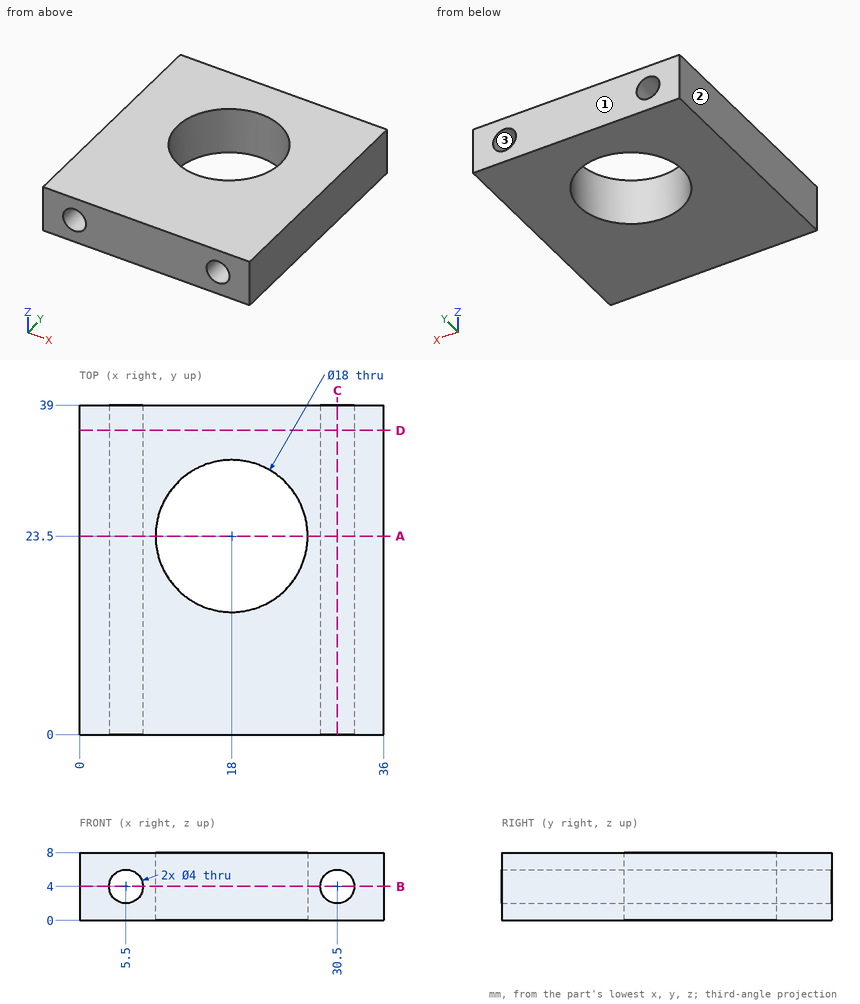
Answer from the drawing. Dimensions are ordinates in mm from the lowest x, y and z of the part. Coordinates: 2 decimals unless noted, no trailing zeros. Order: outer loops, then holes, each group sorted by start corner. A loop starts at its lowest first (then second) coordinate and runs counter-clockwise, first axis right, second up. Notation, with made-up numbers: (19.5, 31.25) - (27.5, 31.25) arc R22 cw to (27.5, 67.25) - close; hole circle Ø4 at (-10, 64.5). An arc over 180 degrees is marked (long way). Answer as a JSON object with one key per item and string values. Group by question number.
Item 1: Section D-D (y = 36) is taken. Give the vertices of the cut face in (x, z).
Item 2: Flat-ended cylindrical pins translate along their axes: P1, Ø1.5, axis at y = 31, z = 5, coming from the -X side; P2, Ø14.5, axis at x = 18, y = 23.5, coming from the +Z side. Find the tip coordinate at first contact, or state that the pin passes through.
Item 3: The mould has two halves that part along X. Classify the marked faces 1, 2 and 3: +X half, -X half, draft (parallel to the pull), parting line (faces both ways), or undercut.
Item 4: Section C-C (x = 30.5) is taken. Give the vertices of the cut face in (y, z).
Item 5: Consider probe 1 along X at (y, z) = (35.5, 4); probe 2 along X at (y, z) = (31.5, 4); probe 3 along X at (y, z) = (30.5, 4). Determine where each line is inside the solid, lowest interval first. Write a range as from..to.
Item 6: Section B-B (z = 4) is taken. Give the vertices of the cut face in (x, y), plus the area to 3 significant figures.
Item 7: Section A-A (y = 23.5) is taken. Give the vertices of the cut face in (x, z), plus the area to 3 significant figures.
Results are:
{
 "1": {"outline": "(0, 0) - (36, 0) - (36, 8) - (0, 8) - close; hole circle Ø4 at (5.5, 4); hole circle Ø4 at (30.5, 4)"},
 "2": {"P1": "stops at x = 0", "P2": "passes through"},
 "3": {"face 1": "draft", "face 2": "-X half", "face 3": "undercut"},
 "4": {"outline": "(0, 0) - (39, 0) - (39, 2) - (0, 2) - close; (0, 6) - (39, 6) - (39, 8) - (0, 8) - close"},
 "5": {"probe 1": "x = 0..3.5, 7.5..28.5, 32.5..36", "probe 2": "x = 0..3.5, 7.5..13.88, 22.12..28.5, 32.5..36", "probe 3": "x = 0..3.5, 7.5..12.34, 23.66..28.5, 32.5..36"},
 "6": {"outline": "(0, 0) - (3.5, 0) - (3.5, 39) - (0, 39) - close; (7.5, 0) - (28.5, 0) - (28.5, 39) - (7.5, 39) - close; (32.5, 0) - (36, 0) - (36, 39) - (32.5, 39) - close; hole circle Ø18 at (18, 23.5)", "area": "838 mm^2"},
 "7": {"outline": "(0, 0) - (9, 0) - (9, 8) - (0, 8) - close; (27, 0) - (36, 0) - (36, 8) - (27, 8) - close; hole circle Ø4 at (5.5, 4); hole circle Ø4 at (30.5, 4)", "area": "119 mm^2"}
}
